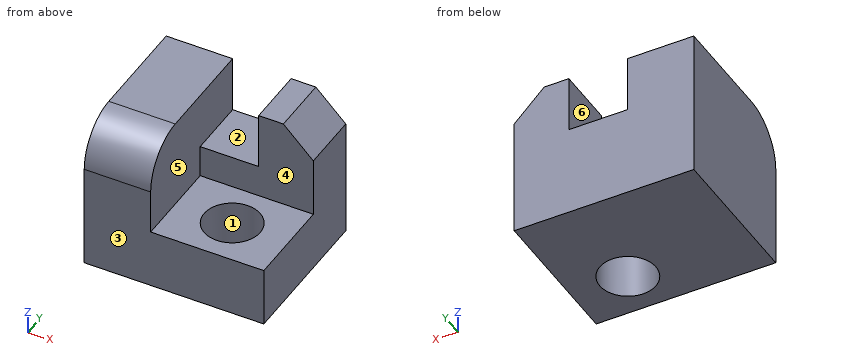
```python
from build123d import *

# Parameters (mm, degrees)
F0_W     = 152.4
F0_H     = 127
F1_DEPTH = 63.5
F2_W     = 96.0077429086
F2_H     = 76.7051585242
F3_DEPTH = 76.2
F4_W     = 49.6507994831
F4_H     = 48.5305104628
F5_DEPTH = 75.184
F6_R     = 38.1
F7_SIZE  = 25.4
F8_R     = 23.7983401661
F9_DEPTH = 86.36


with BuildPart() as f1:
    # F0 (on Front) → F1 (new body, symmetric)
    with BuildSketch(Plane.XZ):
        Rectangle(F0_W, F0_H)
    extrude(amount=F1_DEPTH, both=True)

    # F2 (on face) → F3 (cut)
    with BuildSketch(Plane.XY.offset(63.5)):
        with Locations((28.1961285457, -25.1474207379)):
            Rectangle(F2_W, F2_H)
    extrude(amount=-F3_DEPTH, mode=Mode.SUBTRACT)

    # F4 (on face) → F5 (cut)
    with BuildSketch(Plane.XZ.offset(-13.2051585242)):
        with Locations((5.0176568329, 39.2347447686)):
            Rectangle(F4_W, F4_H)
    extrude(amount=-F5_DEPTH, mode=Mode.SUBTRACT)

    # F6
    f6_edges = [f1.edges().sort_by_distance(p)[0] for p in [
        (-48.003871, -63.5, 63.5),
    ]]
    fillet(f6_edges, radius=F6_R)

    # F7
    f7_edges = [f1.edges().sort_by_distance(p)[0] for p in [
        (76.2, 38.352579, 63.5),
    ]]
    chamfer(f7_edges, length=F7_SIZE)

    # F8 (on face) → F9 (cut)
    with BuildSketch(Plane.XY.offset(-12.7)):
        with Locations((28.1961299479, -24.8870439827)):
            Circle(F8_R)
    extrude(amount=-F9_DEPTH, mode=Mode.SUBTRACT)


solid = f1.part
```
Source: CAD feature listing. Evaluate the final solid. Frame: model axes, mm. Face numbers are marked on the shaded views. A direction names the side the tool comes from. Give positions to 0.01 mm unless a question says otherwise; leave off trailing zeros. Loops run counter-clockwise (first coordinate to the right, second up) from the corner with the lowest first, then second, coordinate; pieces in that order, holes last. Notation, with made-up numbers: (56.25, 4) - (111.25, 4) arc R32 cw to (111.25, 32) - close; hole circle Ø10 at (36.25, -21.5). An arc over 180 degrees is marked (long way). Use CSV: the item, a comma, the result in double quotes.
1) Cut plane D-D (x = -12.5). Output: boundary loops of the cut face in (y, z), and give its area (3 significant figures).
Worked out:
outline,"(-63.5, -63.5) - (63.5, -63.5) - (63.5, 14.97) - (13.21, 14.97) - (13.21, -12.7) - (-63.5, -12.7) - close"
area,"7,840 mm^2"
2) Cut plane B-B (y = 31.5). Output: boundary loops of the cut face in (x, z).
Worked out:
outline,"(-76.2, -63.5) - (76.2, -63.5) - (76.2, 38.1) - (50.8, 63.5) - (29.84, 63.5) - (29.84, 14.97) - (-19.81, 14.97) - (-19.81, 63.5) - (-76.2, 63.5) - close"
3) Mould query, pull axis Y, two halves, no side actions, for the marked faces 1, 2 and 3. Classes: +Y half, -Y half, draft (parallel to the pull), parting line (faces both ways), or undercut.
Worked out:
face 1,"undercut"
face 2,"draft"
face 3,"-Y half"
4) Cut plane A-A (x = 34.5). Output: boundary loops of the cut face in (y, z).
Worked out:
outline,"(-63.5, -63.5) - (-47.84, -63.5) - (-47.84, -12.7) - (-63.5, -12.7) - close; (-1.94, -63.5) - (63.5, -63.5) - (63.5, 63.5) - (13.21, 63.5) - (13.21, -12.7) - (-1.94, -12.7) - close"
5) Cut plane C-C (y = -17). Output: boundary loops of the cut face in (x, z).
Worked out:
outline,"(-76.2, -63.5) - (5.74, -63.5) - (5.74, -12.7) - (-19.81, -12.7) - (-19.81, 63.5) - (-76.2, 63.5) - close; (50.65, -63.5) - (76.2, -63.5) - (76.2, -12.7) - (50.65, -12.7) - close"
6) Pin query (flat end, axial travel): P1, Ø12, axis at x = 14.5, y = 31, coming from the +Z side; P2, Ø6, axis at x = -15.5, y = -21, coming from the +Z side; P3, Ø2, axis at y = -15, z = 18.5, coming from the +X side. Return the tip coordinate at first contact, or that it passes through.
Worked out:
P1,"stops at z = 14.97"
P2,"stops at z = -12.7"
P3,"stops at x = -19.81"
7) Line query: line 1 (X direction, y = -41, z = 9.5); line 2 (Z direction, x = 48.5, y = 3); line 3 (X direction, y = 38.5, z = 22). Output: solid intervals per line, ascending.
Worked out:
line 1,"x = -76.2 to -19.81"
line 2,"z = -63.5 to -12.7"
line 3,"x = -76.2 to -19.81, 29.84 to 76.2"
8) Set-up query: the marked faces 4, 5 and 6. Return all of +Z, -Z, +X, -X, +Y, -Y with unobstructed straight access to the full face (end or side cutting, diameter ignored); none if empty.
Worked out:
face 4,"+Z, +X, -Y"
face 5,"+Z, -Y"
face 6,"+Z, +Y, -Y"
